Build history of the part. All positions in model axes, mm. Give positions to 0.01 mm unless a question says otherwise; leave off trailing zeros. Order: outer loops, then holes, each group sorted by start corner. A loop starts at its lowest first (then second) coordinate and runs counter-clockwise, first axis right, second up. Notation, with made-up numbers: (-12, 44.25) - (43, 44.25) arc R17 cw to (43, 51.25) - close; hole circle Ø10 at (78.5, 34). An arc over 180 degrees is marked (long way). Use a Markdown table: item, result. Add a question column.
(1) Slice it at A-A (y = 0). Write the cut outline in (x, z), then the cut area to 3 significant figures.
(2) Slice it at B-B (z = -2). Write the cut outline in (x, y), then the cut area to 3 significant figures.
(3) Slice it at C-C (x = 0.5). Write the cut outline in (y, z), then the cut area to 3 significant figures.
(4) Flat gauge pins, fed straight in: pin 1 (6 mm diameter, centred on x = 9, z = -0.5, fed in from -Y); pin 2 (1 mm diameter, centred on y = 4.5, z = -3, fed in from +X); pin 3 (1.5 mm diameter, centred on y = -3.5, z = 4.5, fed in from -X). Where does each tip first touch, or does it go through?
(5) Slice it at D-D (x = -7.5). Write the cut outline in (y, z).
(6) Wall check: line 1 (Y direction, x = -6, z = 5); line 2 (X direction, y = 4.75, z = 5.5); line 3 (X direction, y = -1.5, z = 0.5). Give the ranges that are in metal, low to high.
(7) Mould opens along X. For faces 1 (the face through (-1.323, 10.074, -0.089)), 2 (the face through (-5.57, 11.684, 0.09)) say: +X half, -X half, draft (parallel to the pull), parting line (faces both ways), or undercut.
from build123d import *

# Parameters (mm, degrees)
SKETCH1_R           = 11.684
SKETCH1_R_2         = 10.16
BOSS_EXTRUDE1_DEPTH = 6.35
CUT_EXTRUDE1_REACH  = 25.368
SKETCH5_R           = 2.4892


with BuildPart() as part:
    # Sketch1 → Boss-Extrude1 (new body, symmetric)
    with BuildSketch(Plane.XY):
        Circle(SKETCH1_R)
        Circle(SKETCH1_R_2, mode=Mode.SUBTRACT)
        with BuildLine():
            ThreePointArc((-1.880972472, 11.5316), (-0.943568122, 11.645837677), (0, 11.684))
            Line((0, 11.684), (-14.580972472, 11.684))
            Line((-14.580972472, 11.684), (-14.580972472, 11.5316))
            Line((-14.580972472, 11.5316), (-1.880972472, 11.5316))
        make_face()
    extrude(amount=BOSS_EXTRUDE1_DEPTH, both=True)

    # Sketch5 → Cut-Extrude1 (cut, up to next)
    with BuildSketch(Plane(origin=(0, 11.684, 0), x_dir=(1, 0, 0), z_dir=(0, 1, 0)), mode=Mode.PRIVATE) as cut_extrude1_sk1:
        with BuildLine():
            ThreePointArc((-14.580972472, 0), (-14.378526757, 3.200509029), (-13.77441672, 6.35))
            Line((-13.77441672, 6.35), (-14.580972472, 6.35))
            Line((-14.580972472, 6.35), (-14.580972472, 0))
        make_face()
    cut_extrude1_tool1 = extrude(cut_extrude1_sk1.sketch, amount=-CUT_EXTRUDE1_REACH, mode=Mode.PRIVATE) & part.part
    add(cut_extrude1_tool1.solids().sort_by_distance((-14.339679, 11.684, -4.767585))[0], mode=Mode.SUBTRACT)
    # Sketch5 → Cut-Extrude1 (cut, up to next)
    with BuildSketch(Plane(origin=(0, 11.684, 0), x_dir=(1, 0, 0), z_dir=(0, 1, 0)), mode=Mode.PRIVATE) as cut_extrude1_sk2:
        with BuildLine():
            ThreePointArc((-13.77441672, -6.35), (-14.378526757, -3.200509029), (-14.580972472, 0))
            Line((-14.580972472, 0), (-14.580972472, -6.35))
            Line((-14.580972472, -6.35), (-13.77441672, -6.35))
        make_face()
    cut_extrude1_tool2 = extrude(cut_extrude1_sk2.sketch, amount=-CUT_EXTRUDE1_REACH, mode=Mode.PRIVATE) & part.part
    add(cut_extrude1_tool2.solids().sort_by_distance((-14.339679, 11.684, 4.767585))[0], mode=Mode.SUBTRACT)
    # Sketch5 → Cut-Extrude1 (cut, up to next)
    with BuildSketch(Plane(origin=(0, 11.684, 0), x_dir=(1, 0, 0), z_dir=(0, 1, 0)), mode=Mode.PRIVATE) as cut_extrude1_sk3:
        with Locations((-8.230972472, 0)):
            Circle(SKETCH5_R)
    cut_extrude1_tool3 = extrude(cut_extrude1_sk3.sketch, amount=-CUT_EXTRUDE1_REACH, mode=Mode.PRIVATE) & part.part
    add(cut_extrude1_tool3.solids().sort_by_distance((-8.230972, 11.684, 0))[0], mode=Mode.SUBTRACT)


solid = part.part
Solution:
| question | item | result |
|---|---|---|
| 1 | outline | (-11.68, -6.35) - (-10.16, -6.35) - (-10.16, 6.35) - (-11.68, 6.35) - close; (10.16, -6.35) - (11.68, -6.35) - (11.68, 6.35) - (10.16, 6.35) - close |
| 1 | area | 38.7 mm2 |
| 2 | outline | (-14.5, 11.53) - (-9.71, 11.53) - (-9.71, 11.68) - (-14.5, 11.68) - close; (-6.75, 11.53) - (-1.88, 11.53) arc R11.68 ccw (long way) to (0, 11.68) - (-6.75, 11.68) - close; hole circle Ø20.32 at (0, 0) |
| 2 | area | 106 mm2 |
| 3 | outline | (-11.67, -6.35) - (-10.15, -6.35) - (-10.15, 6.35) - (-11.67, 6.35) - close; (10.15, -6.35) - (11.67, -6.35) - (11.67, 6.35) - (10.15, 6.35) - close |
| 3 | area | 38.8 mm2 |
| 4 | pin 1 | y = -10.03 |
| 4 | pin 2 | x = 10.98 |
| 4 | pin 3 | x = -11.36 |
| 5 | outline | (-8.96, -6.35) - (-6.85, -6.35) - (-6.85, 6.35) - (-8.96, 6.35) - close; (6.85, -6.35) - (8.96, -6.35) - (8.96, 6.35) - (6.85, 6.35) - close; (11.53, -6.35) - (11.68, -6.35) - (11.68, -2.38) - (11.53, -2.38) - close; (11.53, 2.38) - (11.68, 2.38) - (11.68, 6.35) - (11.53, 6.35) - close |
| 6 | line 1 | -10.03 to -8.2, 8.2 to 10.03, 11.53 to 11.68 |
| 6 | line 2 | -10.67 to -8.98, 8.98 to 10.67 |
| 6 | line 3 | -11.59 to -10.05, 10.05 to 11.59 |
| 7 | face 1 | undercut |
| 7 | face 2 | draft |
